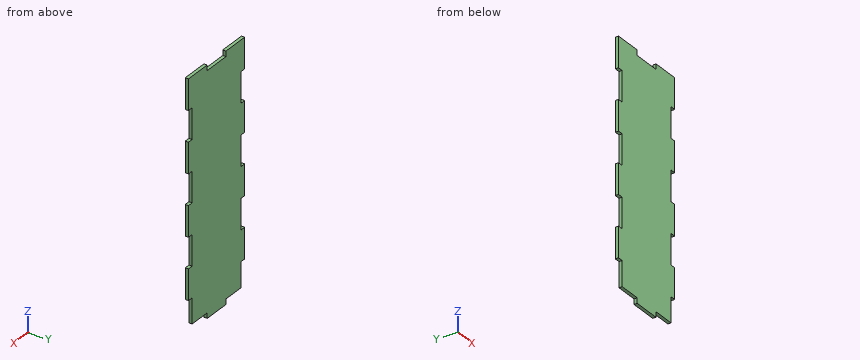
from build123d import *

# Parameters (mm, degrees)
BOSS_EXTRUDE1_DEPTH = 3


with BuildPart() as part:
    # Sketch1 → Boss-Extrude1 (new body)
    with BuildSketch(Plane(origin=(0, 0, 0), x_dir=(1, 0, 0), z_dir=(0, 1, 0))):
        Polygon((-38, -114), (-12.666666667, -114), (-12.666666667, -109), (0, -109), (0, 114), (-12.666666667, 114), (-12.666666667, 109), (-33, 109), (-33, 85.5), (-38, 85.5), (-38, 57), (-33, 57), (-33, 28.5), (-38, 28.5), (-38, 0), (-33, 0), (-33, -28.5), (-38, -28.5), (-38, -57), (-33, -57), (-33, -85.5), (-38, -85.5), align=None)
    boss_extrude1 = extrude(amount=BOSS_EXTRUDE1_DEPTH)

    # Mirror1: Boss-Extrude1 across plane
    add(boss_extrude1.mirror(Plane(origin=(0, 3, 109), x_dir=(0, 0, 1), z_dir=(-1, 0, 0))))


solid = part.part
For this review, take the finished solid that the model builds, in its own axes (mm). Round coordinates to 2 decimals unless told otherwise and drop trailing zeros. Order: outer loops, then holes, each group sorted by start corner. A loop starts at its lowest first (then second) coordinate and runs counter-clockwise, first axis right, second up. Notation, with made-up numbers: (61.25, 23.5) -> (119.25, 23.5) arc R28 ccw to (119.25, 55.5) -> close; hole circle Ø4 at (55, -27). An arc over 180 degrees is marked (long way). Put each result on its own line as item: value.
Q1. Add section A-A on x = -9. Write out the cut boundary in (y, z).
Check result:
outline: (0, -114) -> (3, -114) -> (3, 109) -> (0, 109) -> close
Q2. Insertion check: pin 1 Ø1.5 at (x, y) = (35.5, 2) entering from -Z; pin 2 Ø0.9 at (y, z) = (1, 21) entering from -X; pin 3 Ø0.9 at (y, z) = (2, 76.5) entering from +X; pin 4 Ø8 at (x, z) = (-16, 6.5) entering from -Y. Each pin has a flat end and moves straight along its axis. Give the tip position at first contact, or say it passes through.
Check result:
pin 1: z = -85.5
pin 2: x = -33
pin 3: x = 33
pin 4: y = 0
Q3. Add section B-B on z = 69. Write out the cut boundary in (x, y).
Check result:
outline: (-33, 0) -> (33, 0) -> (33, 3) -> (-33, 3) -> close
Q4. For probe 1 along X at (y, z) = (1.35, 18); probe 2 along Z at (x, y) = (30, 0.95); probe 3 along Z at (x, y) = (10.5, 2), list the stretches that pass through material, from the lowest coordinate up. Write a range as [from, to].
Check result:
probe 1: [-33, 33]
probe 2: [-109, 114]
probe 3: [-114, 109]
